Geometry: see drawing. Coordinates: mm, zero at the bounding-box minimum. A direction names the side the tool comes from. Coordinates: 2 decimals unless noted, no trailing zeros. Order: outer loops, then holes, each group sorted by start corner. A loop starts at its lowest first (then second) coordinate and runs counter-clockwise, first axis right, second up.
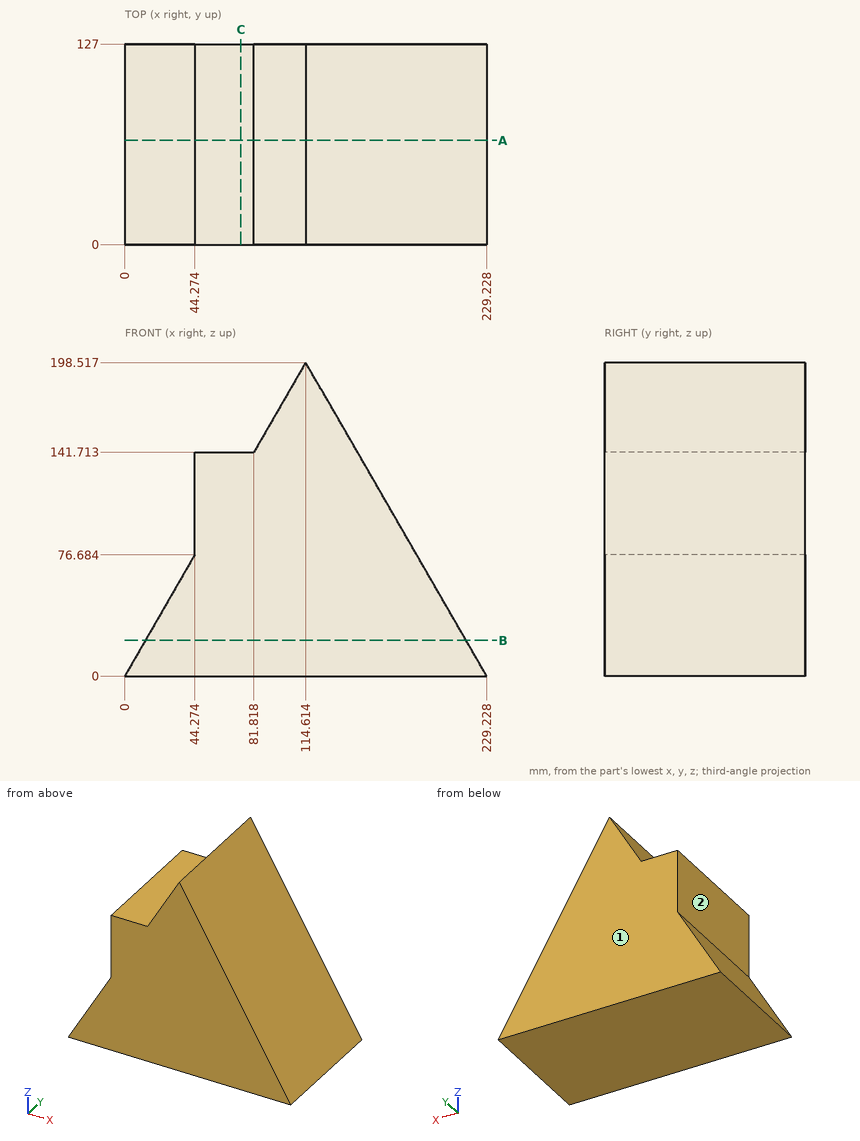
Q1. Section query C-C on x = 73.5. Output: boundary loops of the cut face in (y, z), plus the area to 3 significant figures.
Solutions:
outline: (0, 0) - (127, 0) - (127, 141.71) - (0, 141.71) - close
area: 18,000 mm2
Q2. Section query B-B on z = 22.5. Output: boundary loops of the cut face in (x, y), plus the area to 3 significant figures.
Solutions:
outline: (12.99, 0) - (216.24, 0) - (216.24, 127) - (12.99, 127) - close
area: 25,800 mm2
Q3. Material intervals for line 1 along Z through (x, y) = (65.5, 82.5); line 2 along Z through (x, y) = (170.5, 18); line 3 along X through (y, z) = (67, 95) (1 decimal), sorted ascending.
Solutions:
line 1: z = 0 to 141.71
line 2: z = 0 to 101.72
line 3: x = 44.3 to 174.4
Q4. Section query A-A on y = 66. Output: boundary loops of the cut face in (x, z) (1 decimal), plus the area to 3 significant figures.
Solutions:
outline: (0, 0) - (229.2, 0) - (114.6, 198.5) - (81.8, 141.7) - (44.3, 141.7) - (44.3, 76.7) - close
area: 24,000 mm2
Q5. Set-up query: the marked faces 1 and 2. Return all of +Z, -Z, +X, -X, +Y, -Y with unobstructed straight access to the full face (end or side cutting, diameter ignored); none if empty.
Solutions:
face 1: +Z, -Z, +X, -X, +Y
face 2: +Z, -X, +Y, -Y
Q6. Pin query (flat end, axial travel): P1, Ø11.5, axis at x = 60.5, y = 50, coming from the +Z side; P2, Ø19.5, axis at y = 75, z = 106, coming from the -X side; P3, Ø8, axis at x = 171.5, y = 104.5, coming from the +Z side (1 decimal). Return the tip coordinate at first contact, or that it passes through.
Solutions:
P1: stops at z = 141.71
P2: stops at x = 44.27
P3: stops at z = 106.9
